Could you check a few things on this model? Use its own coordinates, in mm. Coordinates: 2 decimals unless noted, no trailing zeros. Order: outer loops, then holes, each group sorted by start corner. A loop starts at its lowest first (then second) coordinate and runs counter-clockwise, first axis right, second up. Notation, with made-up numbers: (0, -31) -> (26, -31) arc R15 cw to (26, -17) -> close; hole circle Ø1 at (49.25, 42.25). An arc over 180 degrees is marked (long way). Put each result on its own line as item: value. Start each with the question number.
Q1. If we section it at B-B (x = 73): Please give me the cut outline in (y, z).
Q2. Will these pins go through, and if not, where does the flat tip stop? pin 1 (2 mm diameter, centred on x = 44, z = 2, fed in from -Y); pin 2 (1.8 mm diameter, centred on y = 34.5, z = 3, fed in from +X); pin 3 (1.8 mm diameter, centred on x = -104.5, z = 2.5, fed in from -Y).
Q3. If we section it at C-C (y = -55.5): Please give me the cut outline in (x, z).
Q4. If we section it at A-A (z = 2.7): Count the separate pieces of the cut face and the enclosed holes in it, and give its area (3 significant figures).
Q5. Please list where these lines run through material, in increasing order: line 1 along Y through (x, z) = (0, 1.8); line 2 along Y through (x, z) = (-103, 2.15); line 3 along X through (y, z) = (54, 0.9).
Autodesk Inventor part; units mm, degrees
sketch "Sketch1" plane through (0, 0, 0) normal (0, 0, 1) x (1, 0, 0)
  line L0 (-99.5, 74.5) -> (99.5, 74.5)
  line L1 (99.5, 74.5) -> (99.5, -74.5)
  line L2 (99.5, -74.5) -> (-99.5, -74.5)
  line L3 (-99.5, -74.5) -> (-99.5, 74.5)
  point P0 (0, 74.5)
  point P1 (0, 0)
  point P2 (-99.5, 0)
  dimension "d0" = 199
  dimension "d1" = 149
extrude "Extrusion1" add sketch "Sketch1" along normal blind 6
sketch "Sketch2" plane through (0, 0, 6) normal (0, 0, 1) x (1, 0, 0)
  line L0 (-99.5, -74.5) -> (99.5, -74.5)
  line L1 (-99.5, -74.5) -> (-92.5, -74.5)
  line L2 (-92.5, -74.5) -> (-92.5, -67.5)
  line L3 (-92.5, -67.5) -> (-99.5, -67.5)
  line L4 (-99.5, -67.5) -> (-99.5, -74.5)
  point P0 (0, 0)
  point P1 (40.5, -62.5)
  dimension "d18" = 7
  dimension "d19" = 7
extrude "Extrusion2" cut sketch "Sketch2" against normal blind 15
mirror "Mirror3" about plane through (0, 0, 0) normal (1, 0, 0) of "Extrusion2"
mirror "Mirror4" about plane through (0, 0, 0) normal (0, 1, 0) of "Extrusion2", "Mirror3"
sketch "Sketch4" plane through (0, 0, 6) normal (0, 0, 1) x (1, 0, 0)
  line L0 (-99.5, 67.5) -> (-99.5, -67.5)
  line L1 (-99.5, 12.5) -> (-109, 12.5)
  line L2 (-109, 12.5) -> (-109, -12.5)
  line L3 (-109, -12.5) -> (-99.5, -12.5)
  line L4 (-99.5, -12.5) -> (-99.5, 12.5)
  line L5 (-99.5, 0) -> (-103, 0) construction
  circle A0 centre (-103, 0) radius 2.1
  point P0 (0, 0)
  point P1 (-82, 49)
  point P2 (-82, -49)
  point P3 (-99.5, 0)
  point P4 (-99.5, -67.5)
  dimension "d23" = 9.5
  dimension "d24" = 25
  dimension "d34" = 3.5
  dimension "d35" = 4.2
extrude "Extrusion4" add sketch "Sketch4" against normal blind 6
mirror "Mirror5" about plane through (0, 0, 0) normal (1, 0, 0) of "Extrusion4"
sketch "Sketch6" plane through (0, 0, 6) normal (0, 0, 1) x (1, 0, 0)
  line L0 (92.5, 74.5) -> (-92.5, 74.5)
  line L1 (-12.5, 74.5) -> (12.5, 74.5)
  line L2 (12.5, 74.5) -> (12.5, 84)
  line L3 (12.5, 84) -> (-12.5, 84)
  line L4 (-12.5, 84) -> (-12.5, 74.5)
  circle A0 centre (0, 77.5) radius 2.1
  line L5 (0, 74.5) -> (0, 77.5) construction
  point P0 (0, 0)
  dimension "d28" = 25
  dimension "d29" = 9.5
  dimension "d30" = 4.2
  dimension "d36" = 3
extrude "Extrusion5" add sketch "Sketch6" against normal blind 6
mirror "Mirror6" about plane through (0, 0, 0) normal (0, 1, 0) of "Extrusion5"
fillet "Fillet4" radius 1 28 edges at (-109, -12.5, 3) (-99.5, -12.5, 3) (-99.5, -67.5, 3) (-92.5, -67.5, 3) (-92.5, -74.5, 3) (-12.5, -74.5, 3) (-12.5, -84, 3) (12.5, -84, 3) (92.5, -74.5, 3) (99.5, -67.5, 3) (12.5, -74.5, 3) (92.5, -67.5, 3) (99.5, -12.5, 3) (109, -12.5, 3) (109, 12.5, 3) (99.5, 67.5, 3) (92.5, 74.5, 3) (12.5, 84, 3) (92.5, 67.5, 3) (99.5, 12.5, 3) (-12.5, 84, 3) (-92.5, 74.5, 3) (-99.5, 67.5, 3) (-12.5, 74.5, 3) (-92.5, 67.5, 3) (-99.5, 12.5, 3) (-109, 12.5, 3) (12.5, 74.5, 3)
sketch "Sketch7" plane through (0, 0, 6) normal (0, 0, 1) x (1, 0, 0)
  circle A0 centre (0, 0) radius 8.25
  dimension "d38" = 16.5
extrude "Extrusion6" cut sketch "Sketch7" against normal through all
equation "\"d7\" = d5"
properties part number "MDF_Base" material "MDF Medium Density Fiberboard"
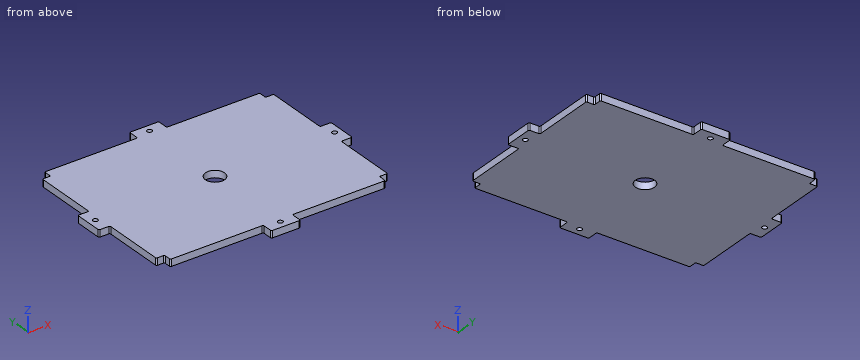
The answers:
1. outline: (-74.5, 0) -> (74.5, 0) -> (74.5, 6) -> (-74.5, 6) -> close
2. pin 1: y = -74.5
2. pin 2: x = 99.5
2. pin 3: y = -12.5
3. outline: (-99.5, 0) -> (99.5, 0) -> (99.5, 6) -> (-99.5, 6) -> close
4. separate pieces: 1
4. enclosed holes: 5
4. area: 30,100 mm^2
5. line 1: -84 to -79.6, -75.4 to -8.25, 8.25 to 75.4, 79.6 to 84
5. line 2: -12.5 to -2.1, 2.1 to 12.5
5. line 3: -99.5 to 99.5
